from build123d import *

# Parameters (mm, degrees)
SKETCH1_R           = 16
SKETCH1_R_2         = 1.75
SKETCH1_R_3         = 11.25
BOSS_EXTRUDE1_DEPTH = 7
SKETCH2_R           = 17.5
BOSS_EXTRUDE2_DEPTH = 108.5
SKETCH3_R           = 4
BOSS_EXTRUDE3_DEPTH = 22.5
BOSS_EXTRUDE4_START = -103.5
SKETCH4_R           = 18
SKETCH4_R_2         = 17.5
BOSS_EXTRUDE4_DEPTH = 58.5
CUT_EXTRUDE1_START  = -8
CUT_EXTRUDE1_DEPTH  = 8
CUT_EXTRUDE3_START  = -8
CUT_EXTRUDE3_DEPTH  = 8


with BuildPart() as part:
    # Sketch1 → Boss-Extrude1 (new body)
    # profile 1 of 2: a face of its own
    with BuildSketch(Plane.XY):
        Circle(SKETCH1_R)
        with Locations((9.899494937, 9.899494937)):
            Circle(SKETCH1_R_2, mode=Mode.SUBTRACT)
        with Locations((-9.899494937, 9.899494937)):
            Circle(SKETCH1_R_2, mode=Mode.SUBTRACT)
        with Locations((-9.899494937, -9.899494937)):
            Circle(SKETCH1_R_2, mode=Mode.SUBTRACT)
        with Locations((9.899494937, -9.899494937)):
            Circle(SKETCH1_R_2, mode=Mode.SUBTRACT)
        Circle(SKETCH1_R_3, mode=Mode.SUBTRACT)
    # profile 2 of 2: a face of its own
    with BuildSketch(Plane.XY):
        Circle(SKETCH1_R_3)
    extrude(amount=BOSS_EXTRUDE1_DEPTH)

    # Sketch2 → Boss-Extrude2 (add)
    with BuildSketch(Plane.XY.offset(7)):
        Circle(SKETCH2_R)
    extrude(amount=BOSS_EXTRUDE2_DEPTH)

    # Sketch3 → Boss-Extrude3 (add)
    with BuildSketch(Plane(origin=(0, 0, 0), x_dir=(-1, 0, 0), z_dir=(0, 0, -1))):
        with Locations(Location((0, 0, 0), (0, 0, 180))):
            Circle(SKETCH3_R)
    extrude(amount=BOSS_EXTRUDE3_DEPTH)

    # Sketch4 → Boss-Extrude4 (add)
    with BuildSketch(Plane.XY.offset(115.5).offset(BOSS_EXTRUDE4_START)):
        Circle(SKETCH4_R)
        Circle(SKETCH4_R_2, mode=Mode.SUBTRACT)
    extrude(amount=BOSS_EXTRUDE4_DEPTH)

    # Sketch5 → Cut-Extrude1 (cut)
    with BuildSketch(Plane.XY.offset(115.5).offset(CUT_EXTRUDE1_START)):
        with BuildLine():
            Line((8, 15.564382416), (8, -15.564382416))
            ThreePointArc((8, -15.564382416), (17.5, 0), (8, 15.564382416))
        make_face()
    extrude(amount=CUT_EXTRUDE1_DEPTH, mode=Mode.SUBTRACT)

    # Sketch6 → Cut-Extrude3 (cut)
    with BuildSketch(Plane.XY.offset(115.5).offset(CUT_EXTRUDE3_START)):
        with BuildLine():
            Line((8, 14.620191517), (8, 15.564382416))
            ThreePointArc((8, 15.564382416), (7.557695982, 15.783891518), (7.109375, 15.990834472))
            ThreePointArc((7.109375, 15.990834472), (5.242211763, 13.802897965), (8, 14.620191517))
        make_face()
        with BuildLine():
            Line((8, -15.564382416), (8, -14.620191517))
            ThreePointArc((8, -14.620191517), (5.242211763, -13.802897965), (7.109375, -15.990834472))
            ThreePointArc((7.109375, -15.990834472), (7.557695982, -15.783891518), (8, -15.564382416))
        make_face()
    extrude(amount=CUT_EXTRUDE3_DEPTH, mode=Mode.SUBTRACT)


solid = part.part
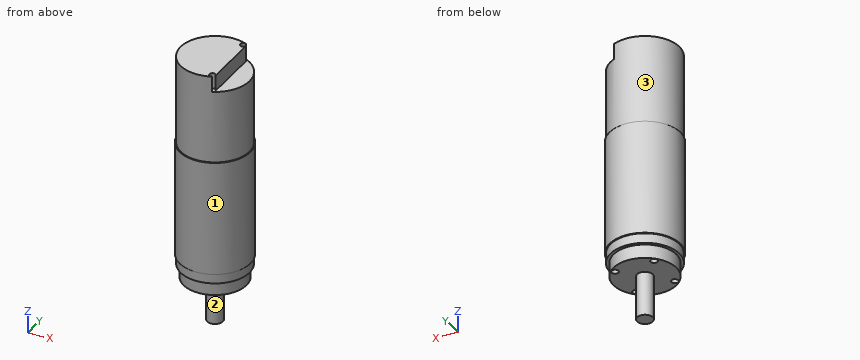
The model under review builds one solid part; all positions refer to its coordinate system, in mm. Face numbers are marked on the shaded views. A direction names the side the tool comes from. Round coordinates to 2 decimals unless told otherwise and drop trailing zeros. Write each loop counter-clockwise with the first axis right and the second up, starting at its lowest first coordinate (ties: lowest second). Pieces come first, ordered by that corner, then holes. Notation, with made-up numbers: M 85.25,65.5 L 138.25,65.5 A27 cw 138.25,88.5 Z; hole C 38.5,-19 d8. An arc over 180 degrees is marked long. Use a Markdown table: item, result. Add a question column.
Q1. We need section C-C, the plane z = 1.5. State the section outline as (x, y) points.
Q2. To check wall thickness, follow line 1 (Y direction, x = 6, z = 112); line 2 (Z direction, x = 6.5, y = 3); line 3 (Z direction, x = 16, y = 5.5). State the ranges of each line that lie inside material, in increasing order.
Q3. We need section B-B, the plane y = 0. State the section outline as (x, z) points, plus the area to 3 significant figures.
Q4. We need section D-D, the plane z = 44. State the section outline as (x, y) points, plus the area to 3 significant figures.
Q5. We need section A-A, the plane x = 0. State the section outline as (y, z) points.
Q6. Machinability: for the marked faces 1, 2 and 3, which of the approach directions +Z, -Z, +X, -X, +Y, -Y give a long, thin tool a straight path to every point of the face, cutting with its end or side? Answer none if there is none.
Q7. Insertion check: pin 1 (5 mm diameter, centred on x = 6.5, y = 14.62, fed in from -Z); pin 2 (2 mm diameter, centred on x = 1, z = 0.5, fed in from +Y); pin 3 (4 mm diameter, centred on y = 4, z = 52, fed in from +X). Each pin has a flat end and moves straight along its axis. Give the tip position at first contact, or say it passes through.
Findings below:
| question | item | result |
|---|---|---|
| 1 | outline | C 0,0 d32; hole C -9.9,-9.9 d3.5; hole C -9.9,9.9 d3.5; hole C 9.9,-9.9 d3.5; hole C 9.9,9.9 d3.5 |
| 2 | line 1 | y = -16.44 to -16.03, -13.21 to 13.21, 16.03 to 16.44 |
| 2 | line 2 | z = 0 to 115.5 |
| 2 | line 3 | z = 7 to 107.5 |
| 3 | outline | M -18,12 L -17.5,12 L -17.5,7 L -16,7 L -16,0 L -4,0 L -4,-22.5 L 4,-22.5 L 4,0 L 16,0 L 16,7 L 17.5,7 L 17.5,12 L 18,12 L 18,70.5 L 17.5,70.5 L 17.5,107.5 L 8,107.5 L 8,115.5 L -17.5,115.5 L -17.5,70.5 L -18,70.5 Z |
| 3 | area | 4,180 mm² |
| 4 | outline | C 0,0 d36 |
| 4 | area | 1,020 mm² |
| 5 | outline | M -18,12 L -17.5,12 L -17.5,7 L -16,7 L -16,0 L -4,0 L -4,-22.5 L 4,-22.5 L 4,0 L 16,0 L 16,7 L 17.5,7 L 17.5,12 L 18,12 L 18,70.5 L 17.5,70.5 L 17.5,115.5 L -17.5,115.5 L -17.5,70.5 L -18,70.5 Z |
| 6 | face 1 | +Z, -Z |
| 6 | face 2 | -Z |
| 6 | face 3 | +Z |
| 7 | pin 1 | stops at z = 0 |
| 7 | pin 2 | stops at y = 16 |
| 7 | pin 3 | stops at x = 17.89 |
